For this review, take the finished solid that the model builds, in its own axes (mm). Face numbers are marked on the shaded views. A direction names the side the tool comes from. Round coordinates to 2 decimals unless told otherwise and drop trailing zeros. Order: outer loops, then holes, each group sorted by start corner. A loop starts at its lowest first (then second) coordinate and runs counter-clockwise, first axis right, second up. Notation, with made-up numbers: M -12.5,-7.5 L 42.5,-7.5 A25 ccw 42.5,6.5 Z; hole C 43.25,-33.75 d6. An arc over 180 degrees is marked long. Answer in a Markdown table with one row per item. Add a question column.
Autodesk Inventor part; units mm, degrees
ref_plane "Work Plane1" through (0, 0, 0) normal (0, 0, 1) x (1, 0, 0)
ref_plane "YZ Plane" through (0, 0, 0) normal (1, 0, 0) x (0, 1, 0)
ref_plane "XZ Plane" through (0, 0, 0) normal (0, 1, 0) x (-1, 0, 0)
ref_plane "Work Plane1" through (0, 0, 0) normal (0, 0, 1) x (1, 0, 0)
sketch "Sketch1" plane through (0, 0, 0) normal (0, 0, 1) x (1, 0, 0)
  line L0 (-135, 150) -> (-135, -150)
  arc A0 (-135, -150) -> (135, -150) centre (0, -150) ccw
  line L1 (135, -150) -> (135, 150)
  arc A1 (135, 150) -> (-135, 150) centre (0, 150) ccw
  line L2 (-80, -150) -> (-80, 150)
  arc A2 (80, 150) -> (-80, 150) centre (0, 150) ccw
  line L3 (80, 150) -> (80, -150)
  arc A3 (-80, -150) -> (80, -150) centre (0, -150) ccw
  line L4 (0, 0) -> (-135, 0)
  line L5 (0, 0) -> (0, 285)
  line L6 (-75, 150) -> (-75, -150)
  arc A4 (-75, -150) -> (75, -150) centre (0, -150) ccw
  line L7 (75, -150) -> (75, 150)
  arc A5 (75, 150) -> (-75, 150) centre (0, 150) ccw
  point P0 (0, 230)
  point P1 (-80, 0)
  point P2 (0, 225)
  point P3 (-75, 0)
  point P4 (135, 0)
  point P5 (-75, 0)
  point P6 (0, -230)
  dimension "d18" = 5
  dimension "d34" = 300
  dimension "d37" = 55
  dimension "d38" = 75
  dimension "d39" = 75
extrude "Extrusion1" add sketch "Sketch1" along normal blind 3 contours A1 L5 A2 L2 L4 L0 | L2 A2 L5 A5 L6 L4
sketch "Sketch2" plane through (0, 0, 3) normal (0, 0, 1) x (1, 0, 0)
  arc A0 (0, 285) -> (-135, 150) centre (0, 150) ccw
  line L0 (-135, 150) -> (-135, 0)
  line L1 (-135, 0) -> (-75, 0) construction
  line L2 (0, 225) -> (0, 285) construction
  line L3 (-75, 0) -> (-75, 150)
  arc A1 (0, 225) -> (-75, 150) centre (0, 150) ccw
  point P0 (0, 0)
sketch "Sketch3" plane through (-135, 0, 0) normal (0, -1, 0) x (1, 0, 0)
  line L0 (0, 0) -> (-13, 0)
  line L1 (-13, 0) -> (-13, 6.35)
  line L2 (-13, 6.35) -> (0, 6.35)
  line L3 (0, 6.35) -> (0, 0)
  circle A0 centre (-6.5, 6.35) radius 4.7625 construction
  line L4 (-11.2625, 11.1125) -> (-1.7375, 11.1125)
  line L5 (-1.7375, 11.1125) -> (-1.7375, 1.5875)
  line L6 (-1.7375, 1.5875) -> (-11.2625, 1.5875)
  line L7 (-11.2625, 1.5875) -> (-11.2625, 11.1125)
  line L8 (-11.2625, 11.1125) -> (-1.7375, 1.5875) construction
  line L9 (-1.7375, 11.1125) -> (-11.2625, 1.5875) construction
  point P0 (135, 0)
  point P1 (-1.7375, 6.35)
  point P2 (-11.2625, 6.35)
  point P3 (-1.7375, 6.35)
  point P4 (-11.2625, 6.35)
  dimension "d2" = 13
  dimension "d3" = 6.35
  dimension "d4" = 9.525
  dimension "d5" = 0
sweep "Sweep1" add profiles "Sketch3" path "Sketch2" path curves L0 A0 contours L0 L1 L2 L7 L6 L5 L3
sketch "Sketch6" plane through (-75, 0, 0) normal (0, -1, 0) x (1, 0, 0)
  arc A0 (-63.7625, 6.35) -> (-54.2375, 6.35) centre (-59, 6.35) ccw
  circle A1 centre (-59, 6.35) radius 4.7625
  circle A2 centre (-59, 6.35) radius 3.175
  point P0 (75, 0)
  point P1 (-54.2375, 6.35)
  dimension "d14" = 9.525
  dimension "d15" = 6.35
sketch3d "3D Sketch1"
sweep "Sweep2" [suppressed]
sketch "Sketch4" plane through (0, 0, 3) normal (0, 0, 1) x (1, 0, 0)
  line L0 (0, 0) -> (-148.7625, 0)
  line L1 (-148.7625, 0) -> (-148.7625, 20)
  line L2 (-148.7625, 20) -> (0, 20)
  line L3 (0, 20) -> (0, 0)
  line L4 (0, 0) -> (-20, 0)
  line L5 (-20, 0) -> (-20, 308)
  line L6 (-20, 308) -> (0, 308)
  line L7 (0, 308) -> (0, 0)
  line L8 (-138.7625, 0) -> (-138.7625, 300)
  point P0 (0, 298)
  point P1 (-20, 20)
  point P2 (-138.7625, 20)
  dimension "d8" = 20
  dimension "d9" = 20
  dimension "d10" = 10
  dimension "d11" = 10
extrude "Extrusion2" cut sketch "Sketch4" against normal through all both and the other way through all contours L0 L8 L2 L5 | L2 L5 L6 L7 | L0 L1 L2 L8 bodies 1
sketch "Sketch7" plane through (0, 0, 3) normal (0, 0, 1) x (1, 0, 0)
  line L0 (-20, 222.2842) -> (-20, 283.5103)
  arc A0 (-20, 283.5103) -> (-135, 150) centre (0, 150) ccw
  line L1 (-135, 150) -> (-135, 0)
  line L2 (-135, 20) -> (-75, 20)
  line L3 (-75, 20) -> (-75, 150)
  arc A1 (-20, 222.2842) -> (-75, 150) centre (0, 150) ccw
  line L4 (-78.5, 150) -> (-78.5, 23.5)
  line L5 (-78.5, 23.5) -> (-131.5, 23.5)
  line L6 (-131.5, 23.5) -> (-131.5, 150)
  arc A2 (-23.5, 279.3832) -> (-131.5, 150) centre (0, 150) ccw
  line L7 (-23.5, 279.3832) -> (-23.5, 224.8999)
  arc A3 (-23.5, 224.8999) -> (-78.5, 150) centre (0, 150) ccw
  point P0 (0, 0)
  point P1 (-131.5, 33.5)
  point P2 (-127.5939, 181.8127)
  point P3 (-116.1076, 211.7355)
  point P4 (-97.7235, 237.9907)
  point P5 (-73.5339, 259.0184)
  point P6 (-44.9756, 273.5696)
  point P7 (-131.5, 66.5)
  point P8 (-131.5, 99.5)
  point P9 (-131.5, 132.5)
  dimension "d21" = 3.5
  dimension "d24" = 70
  dimension "d26" = 10
  dimension "d29" = 33
hole "Hole1" at (-131.5, 33.5, 3) at (-131.5, 150, 3) at (-127.5939, 181.8127, 3) at (-116.1076, 211.7355, 3) at (-97.7235, 237.9907, 3) at (-73.5339, 259.0184, 3) at (-44.9756, 273.5696, 3) at (-131.5, 66.5, 3) at (-131.5, 99.5, 3) at (-131.5, 132.5, 3) direction (0, 0, -1) diameter 3.4 end through all bodies 1
fillet "Fillet1" radius 10 1 edges at (-75, 20, 1.5)
sketch "Sketch8" plane through (0, 0, 3) normal (0, 0, 1) x (1, 0, 0)
  arc A0 (-85, 20) -> (-75, 30) centre (-85, 30) ccw
  line L0 (-75, 30) -> (-75, 150)
  arc A1 (-20, 222.2842) -> (-75, 150) centre (0, 150) ccw
  line L1 (-20, 222.2842) -> (-20, 283.5103)
  arc A2 (-20, 283.5103) -> (-135, 150) centre (0, 150) ccw
  line L2 (-135, 150) -> (-135, 20)
  line L3 (-135, 20) -> (-85, 20)
  line L4 (-74.9, 150) -> (-74.9, 30)
  arc A3 (-85, 19.9) -> (-74.9, 30) centre (-85, 30) ccw
  line L5 (-85, 19.9) -> (-135.1, 19.9)
  line L6 (-135.1, 19.9) -> (-135.1, 150)
  arc A4 (-19.9, 283.6263) -> (-135.1, 150) centre (0, 150) ccw
  line L7 (-19.9, 283.6263) -> (-19.9, 222.208)
  arc A5 (-19.9, 222.208) -> (-74.9, 150) centre (0, 150) ccw
  point P0 (0, 0)
  dimension "d48" = 0.1
extrude "Extrusion3" [suppressed]
sketch "Sketch11" plane through (0, 0, 3) normal (0, 0, 1) x (1, 0, 0)
  line L0 (-135, 150) -> (-135, 20)
  circle A0 centre (-131.5, 99.5) radius 1.7
  circle A1 centre (-44.9756, 273.5696) radius 1.7
  circle A2 centre (-97.7235, 237.9907) radius 1.7
  circle A3 centre (-127.5939, 181.8127) radius 1.7
  circle A4 centre (-131.5, 33.5) radius 1.7
  circle A5 centre (-131.5, 150) radius 1.7
  circle A6 centre (-116.1076, 211.7355) radius 1.7
  circle A7 centre (-73.5339, 259.0184) radius 1.7
  circle A8 centre (-131.5, 66.5) radius 1.7
  circle A9 centre (-131.5, 132.5) radius 1.7
  line L1 (-20, 277.0859) -> (-20, 222.2842)
  arc A10 (-20, 222.2842) -> (-75, 150) centre (0, 150) ccw
  arc A11 (-23, 224.5319) -> (-78, 150) centre (0, 150) ccw
  line L2 (-23, 224.5319) -> (-23, 276.5773)
  line L3 (-135, 20) -> (-85, 20)
  line L4 (-128.65, 20) -> (-85, 20)
  arc A12 (-85, 20) -> (-75, 30) centre (-85, 30) ccw
  arc A13 (-85, 23) -> (-78, 30) centre (-85, 30) ccw
  line L5 (-85, 23) -> (-131.0405, 23)
  line L6 (-78, 150) -> (-78, 30)
  arc A14 (-85, 20) -> (-75, 30) centre (-85, 30) ccw
  line L7 (-75, 30) -> (-75, 150)
  line L8 (-20, 222.2842) -> (-20, 283.5103)
  arc A15 (-20, 283.5103) -> (-135, 150) centre (0, 150) ccw
  point P0 (0, 0)
  dimension "d53" = 3
  dimension "d54" = 3
sketch "Sketch12" plane through (0, 0, 3) normal (0, 0, 1) x (1, 0, 0)
  arc A0 (-85, 20) -> (-75, 30) centre (-85, 30) ccw
  line L0 (-75, 30) -> (-75, 150)
  arc A1 (-20, 222.2842) -> (-75, 150) centre (0, 150) ccw
  line L1 (-20, 222.2842) -> (-20, 283.5103)
  arc A2 (-20, 283.5103) -> (-135, 150) centre (0, 150) ccw
  line L2 (-135, 150) -> (-135, 20)
  line L3 (-135, 20) -> (-85, 20)
  circle A3 centre (-131.5, 99.5) radius 1.7
  circle A4 centre (-44.9756, 273.5696) radius 1.7
  circle A5 centre (-97.7235, 237.9907) radius 1.7
  circle A6 centre (-127.5939, 181.8127) radius 1.7
  circle A7 centre (-131.5, 33.5) radius 1.7
  circle A8 centre (-131.5, 150) radius 1.7
  circle A9 centre (-116.1076, 211.7355) radius 1.7
  circle A10 centre (-73.5339, 259.0184) radius 1.7
  circle A11 centre (-131.5, 66.5) radius 1.7
  circle A12 centre (-131.5, 132.5) radius 1.7
  point P0 (0, 0)
  point P1 (-106.1535, 4.76)
  point P2 (-134.9295, 287.3233)
  dimension "d55" = 15.24
fillet "Fillet2" radius 4.7625 4 edges at (-110.2678, 246.0923, 1.5875) (-146.2625, 85, 1.5875) (-103.5179, 239.3375, 1.5875) (-136.7375, 85, 1.5875)
equation "\"d39\" = d38"
properties part number "1122_Middle Heat Sink_V1" material "Aluminum 6061"
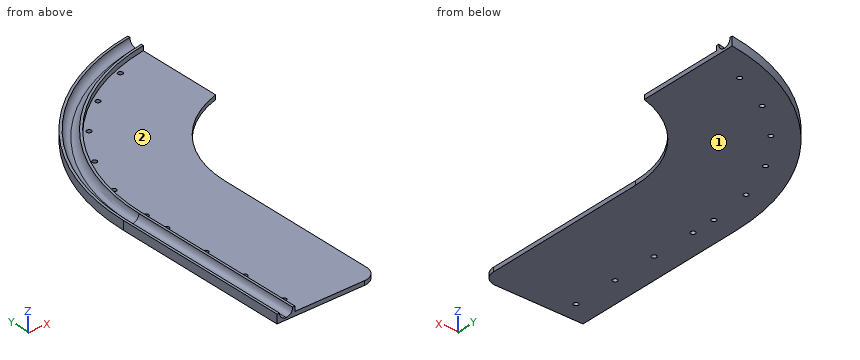
1. For the marked faces 1 and 2, list the 3-axis set-ups (+Z, -Z, +X, -X, +Y, -Y) from which the entire face can be reached by the end or side of a thin tool; tool diameter is ignored.
2. Consider section A-A on z = 4.5. Write out the cut boundary in (x, y).
3. Clearance check with flat-ended pins moving along their axes: pin 1 Ø3 at (x, z) = (-79.5, 1.5) entering from -Y; pin 2 Ø6 at (x, y) = (-107, 183.5) entering from +Z; pin 3 Ø3 at (x, z) = (-51.5, 3) entering from +Y. State where each tip first meets the part, or that it passes through.
4. To check wall thickness, follow probe 1 along Z at (x, y) = (-97, 136); probe 2 along X at (y, z) = (66.5, 0.6); probe 3 along X at (y, z) = (161, 5). State the ranges of each line that lie inside material, in increasing order. Write a range as [from, to].
Solved:
| question | item | result |
|---|---|---|
| 1 | face 1 | -Z, +X, -X, +Y, -Y |
| 1 | face 2 | +Z, +X, -Y |
| 2 | outline | M -148,20 L -145.89,20 L -145.89,150 A145.89 cw -20,294.51 L -20,296.64 A148 ccw -148,150 Z; M -137.11,20 L -135,20 L -135,150 A135 cw -20,283.51 L -20,285.64 A137.11 ccw -137.11,150 Z |
| 3 | pin 1 | stops at y = 20.83 |
| 3 | pin 2 | stops at z = 3 |
| 3 | pin 3 | stops at y = 289.3 |
| 4 | probe 1 | z = [0, 3] |
| 4 | probe 2 | x = [-148, -133.2], [-129.8, -75] |
| 4 | probe 3 | x = [-147.59, -145.65], [-136.49, -134.55] |
